Model file for the job. Use its own axes, mm. Face numbers are marked on the shaded views. Give positions to 0.01 mm unless a question says otherwise; leave off trailing zeros. Order: outer loops, then holes, each group sorted by start corner. A loop starts at its lowest first (then second) coordinate and runs counter-clockwise, first axis right, second up. Notation, with made-up numbers: (24, 34.25) - (36, 34.25) arc R19 ccw to (36, 45.25) - close; hole circle Ø2 at (-14.5, 13.5). An arc over 180 degrees is marked (long way). Use CSV: the item, a comma, the result in double quotes. Start each with the question number.
(1) Probe L1, parallel to Z at x = 0, y = 1.55; L2, parallel to X at y = 1.55, z = 317.5; L3, parallel to X at y = 9.25, z = 299.5. List the from-to ranges inside material, lowest first.
(2) Band-saw the part on A-A, the plane y = 10. Give the cut face in (x, z), then the cut area to 3 significant figures.
(3) Drop flat-ended pins along their axis: pin 1 Ø6 at (x, z) = (-10.5, 104) entering from +Y; pin 2 Ø8 at (x, z) = (0, 12.7) entering from +Y. Give the stop position or say it passes through.
(4) Band-saw the part on B-B, the plane z = 76.5. Give the cut face in (x, y).
(5) Pull direction X, two halves, no side cores. Call the marked faces 1 and 2: +X half, -X half, draft (parallel to the pull), parting line (faces both ways), or undercut.
from build123d import *

# Parameters (mm, degrees)
BOSS_EXTRUDE1_DEPTH                           = 457.2
CSK_FOR_1_4_FLAT_HEAD_MACHINE_SCREW3_AT_COUNT = 2
CSK_FOR_1_4_FLAT_HEAD_MACHINE_SCREW3_AT_PITCH = 76.2
CSK_FOR_1_4_FLAT_HEAD_MACHINE_SCREW3_2_COUNT  = 2
CSK_FOR_1_4_FLAT_HEAD_MACHINE_SCREW3_2_PITCH  = 152.4
CSK_FOR_1_4_FLAT_HEAD_MACHINE_SCREW3_3_COUNT  = 2
CSK_FOR_1_4_FLAT_HEAD_MACHINE_SCREW3_3_PITCH  = 228.6
CSK_FOR_1_4_FLAT_HEAD_MACHINE_SCREW3_4_COUNT  = 2
CSK_FOR_1_4_FLAT_HEAD_MACHINE_SCREW3_4_PITCH  = 304.8


with BuildPart() as part:
    # Sketch → Boss-Extrude1 (new body)
    with BuildSketch(Plane.XY):
        Polygon((-17.78, 6.35), (-17.78, 12.7), (-25.4, 12.7), (-25.4, 0), (25.4, 0), (25.4, 12.7), (17.78, 12.7), (17.78, 6.35), align=None)
    extrude(amount=BOSS_EXTRUDE1_DEPTH)

    # Sketch4 → CSK for 1/4 Flat Head Machine Screw3 (revolve, cut)
    with BuildSketch(Plane(origin=(0, 6.35, 12.7), x_dir=(0, 0, 1), z_dir=(1, 0, 0))):
        Polygon((0, 0), (0, 6.35), (3.3782, 6.35), (3.3782, 4.28291499), (7.1012812, 0), align=None)
    csk_for_1_4_flat_head_machine_screw3 = revolve(axis=Axis((0, 12.7, 12.7), (0, -1, 0)), mode=Mode.SUBTRACT)

    # CSK for 1/4 Flat Head Machine Screw3 at: CSK for 1/4 Flat Head Machine Screw3 ×2
    with Locations(*[(0, 0, i * CSK_FOR_1_4_FLAT_HEAD_MACHINE_SCREW3_AT_PITCH) for i in range(1, CSK_FOR_1_4_FLAT_HEAD_MACHINE_SCREW3_AT_COUNT)]):
        add(csk_for_1_4_flat_head_machine_screw3, mode=Mode.SUBTRACT)

    # CSK for 1_4 Flat Head Machine Screw3 2: CSK for 1/4 Flat Head Machine Screw3 ×2
    with Locations(*[(0, 0, i * CSK_FOR_1_4_FLAT_HEAD_MACHINE_SCREW3_2_PITCH) for i in range(1, CSK_FOR_1_4_FLAT_HEAD_MACHINE_SCREW3_2_COUNT)]):
        add(csk_for_1_4_flat_head_machine_screw3, mode=Mode.SUBTRACT)

    # CSK for 1_4 Flat Head Machine Screw3 3: CSK for 1/4 Flat Head Machine Screw3 ×2
    with Locations(*[(0, 0, i * CSK_FOR_1_4_FLAT_HEAD_MACHINE_SCREW3_3_PITCH) for i in range(1, CSK_FOR_1_4_FLAT_HEAD_MACHINE_SCREW3_3_COUNT)]):
        add(csk_for_1_4_flat_head_machine_screw3, mode=Mode.SUBTRACT)

    # CSK for 1_4 Flat Head Machine Screw3 4: CSK for 1/4 Flat Head Machine Screw3 ×2
    with Locations(*[(0, 0, i * CSK_FOR_1_4_FLAT_HEAD_MACHINE_SCREW3_4_PITCH) for i in range(1, CSK_FOR_1_4_FLAT_HEAD_MACHINE_SCREW3_4_COUNT)]):
        add(csk_for_1_4_flat_head_machine_screw3, mode=Mode.SUBTRACT)


solid = part.part
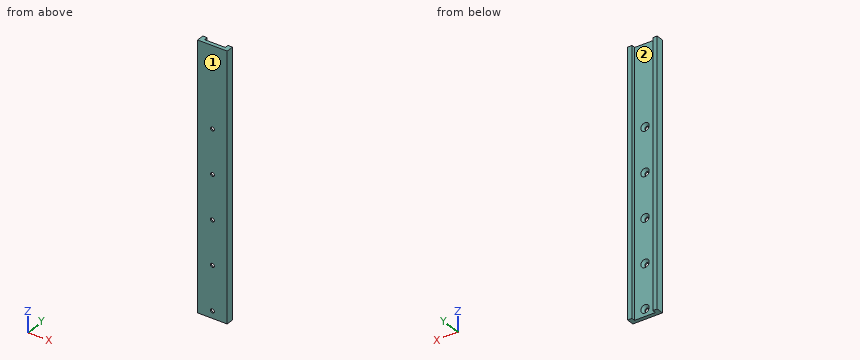
Answer block:
1,L1,"z = 0 to 9.32, 16.08 to 85.52, 92.28 to 161.72, 168.48 to 237.92, 244.68 to 314.12, 320.88 to 457.2"
1,L2,"x = -25.4 to -3.38, 3.38 to 25.4"
1,L3,"x = -25.4 to -17.78, 17.78 to 25.4"
2,outline,"(-25.4, 0) - (-17.78, 0) - (-17.78, 457.2) - (-25.4, 457.2) - close; (17.78, 0) - (25.4, 0) - (25.4, 457.2) - (17.78, 457.2) - close"
2,area,"6,970 mm2"
3,pin 1,"stops at y = 6.35"
3,pin 2,"stops at y = 2.78"
4,outline,"(-25.4, 0) - (25.4, 0) - (25.4, 12.7) - (17.78, 12.7) - (17.78, 6.35) - (-17.78, 6.35) - (-17.78, 12.7) - (-25.4, 12.7) - close"
5,face 1,"draft"
5,face 2,"undercut"
